```python
from build123d import *

# Parameters (mm, degrees)
BOSS_EXTRUDE1_DEPTH = 3


with BuildPart() as part:
    # Sketch2 → Boss-Extrude1 (new body)
    with BuildSketch(Plane(origin=(0, 0, 0), x_dir=(0, 0, -1), z_dir=(1, 0, 0))):
        Polygon((0.000317111, 27.796332929), (0.000317111, 29.796332929), (-3.999682889, 29.796332929), (-6.999682889, 29.796332929), (-6.999682889, 27.796332929), align=None)
        Polygon((-6.999682889, 29.796332929), (-3.999682889, 29.796332929), (-5.499682889, 31.296332929), align=None)
    extrude(amount=BOSS_EXTRUDE1_DEPTH)


solid = part.part
```
Here's how the part is built. I have some questions about the finished solid (model axes, mm). A direction names the side the tool comes from. Round coordinates to 2 decimals unless told otherwise and drop trailing zeros. Order: outer loops, then holes, each group sorted by start corner. A loop starts at its lowest first (then second) coordinate and runs counter-clockwise, first axis right, second up. Notation, with made-up numbers: M -28,-4.75 L 0,-4.75 A31 cw 0,34.25 Z; hole C -34,29 d8. An arc over 180 degrees is marked long. Answer as CSV lines item,"result".
Item 1: Please list where these lines run through material, in increasing order: L1, parallel to Y at x = 2.1, z = 3.25; L2, parallel to Z at x = 2.65, y = 31; L3, parallel to Y at x = 2.6, z = 5. Write a range as [from, to].
From the geometry:
L1,"[27.8, 29.8]"
L2,"[5.2, 5.8]"
L3,"[27.8, 30.8]"
Item 2: Imagine slicing it at B-B on z = 3.75. List the corners of the cut face in (x, y) for me, and give its area (3 significant figures).
From the geometry:
outline,"M 0,27.8 L 3,27.8 L 3,29.8 L 0,29.8 Z"
area,"6.00 mm2"
Item 3: Imagine slicing it at C-C on y = 30.75. List the corners of the cut face in (x, z) for me, and give its area (3 significant figures).
From the geometry:
outline,"M 0,4.95 L 3,4.95 L 3,6.05 L 0,6.05 Z"
area,"3.28 mm2"
Item 4: Imagine slicing it at A-A on x = 0.4. List the corners of the cut face in (y, z) for me, and give its area (4 significant figures).
From the geometry:
outline,"M 27.8,0 L 29.8,0 L 29.8,4 L 31.3,5.5 L 29.8,7 L 27.8,7 Z"
area,"16.25 mm2"
Item 5: For pin 1 (0.9 mm diameter, centred on x = 1.5, z = 1.5, fed in from +Y), with a flat end and sliding along its axis, tell me the tip position at first contact or that it passes through.
From the geometry:
pin 1,"y = 29.8"
Item 6: Which directions (+Z, -Z, +X, -X, +Y, -Y) give clear straight access to the entire face, cutting with the end or side of a thin tool? Please do faces 1 (the flat face through (1, 29.796, 2)), 2 (the flat face through (1, 29, 7)).
From the geometry:
face 1,"-Z, +X, -X, +Y"
face 2,"+Z, +X, -X, +Y, -Y"
